from build123d import *

# Parameters (mm, degrees)
SKETCH_1_W                 = 140
SKETCH_1_H                 = 120
SKETCH_1_R                 = 11.5
EXTRUDE_1_DEPTH            = 4
SKETCH_31_R                = 2.05
SKETCH_31_R_2              = 2.1
CUT_EXTRUDE_16_DEPTH       = 10
MIRROR_2_COPY_1_SKETCH_R   = 2.05
MIRROR_2_COPY_1_SKETCH_R_2 = 2.1
MIRROR_2_COPY_1_DEPTH      = 10
FILLET_8_R                 = 25
SKETCH_32_R                = 2.1
CUT_EXTRUDE_17_DEPTH       = 10
SKETCH_33_R                = 1.6
CUT_EXTRUDE_18_DEPTH       = 10


with BuildPart() as part:
    # 草图1 → 凸台-拉伸1 (new body)
    with BuildSketch(Plane.XY):
        with Locations((70, 60)):
            Rectangle(SKETCH_1_W, SKETCH_1_H)
        with Locations((70, 60)):
            Circle(SKETCH_1_R, mode=Mode.SUBTRACT)
    extrude(amount=EXTRUDE_1_DEPTH)

    # 草图31 → 切除-拉伸16 (cut)
    with BuildSketch(Plane.XY.offset(4)):
        with Locations((9, 60)):
            Circle(SKETCH_31_R)
        with Locations((9, 88)):
            Circle(SKETCH_31_R_2)
    cut_extrude_16 = extrude(amount=-CUT_EXTRUDE_16_DEPTH, mode=Mode.SUBTRACT)

    # 镜向1: 切除-拉伸16 across plane
    add(cut_extrude_16.mirror(Plane.ZX.offset(60)), mode=Mode.SUBTRACT)

    # 镜向2: 切除-拉伸16 across plane
    add(cut_extrude_16.mirror(Plane.ZY.offset(-70)), mode=Mode.SUBTRACT)

    # 镜向2 copy 1 sketch → 镜向2 copy 1 (cut)
    with BuildSketch(Plane(origin=(140, 120, 4), x_dir=(-1, 0, 0), z_dir=(0, 0, 1))):
        with Locations((9, 60)):
            Circle(MIRROR_2_COPY_1_SKETCH_R)
        with Locations((9, 88)):
            Circle(MIRROR_2_COPY_1_SKETCH_R_2)
    extrude(amount=-MIRROR_2_COPY_1_DEPTH, mode=Mode.SUBTRACT)

    # 圆角8
    fillet_8_edges = [part.edges().sort_by_distance(p)[0] for p in [
        (0, 120, 2),
        (140, 120, 2),
        (140, 0, 2),
        (0, 0, 2),
    ]]
    fillet(fillet_8_edges, radius=FILLET_8_R)

    # 草图32 → 切除-拉伸17 (cut)
    with BuildSketch(Plane.XY.offset(4)):
        with Locations((70, 112.5)):
            Circle(SKETCH_32_R)
        with Locations((107.123106012, 97.123106012)):
            Circle(SKETCH_32_R)
        with Locations((122.5, 60)):
            Circle(SKETCH_32_R)
        with Locations((107.123106012, 22.876893988)):
            Circle(SKETCH_32_R)
        with Locations((70, 7.5)):
            Circle(SKETCH_32_R)
        with Locations((32.876893988, 22.876893988)):
            Circle(SKETCH_32_R)
        with Locations((17.5, 60)):
            Circle(SKETCH_32_R)
        with Locations((32.876893988, 97.123106012)):
            Circle(SKETCH_32_R)
    extrude(amount=-CUT_EXTRUDE_17_DEPTH, mode=Mode.SUBTRACT)

    # 草图33 → 切除-拉伸18 (cut)
    with BuildSketch(Plane.XY.offset(4)):
        with Locations((70, 80)):
            Circle(SKETCH_33_R)
        with Locations((87.320508076, 50)):
            Circle(SKETCH_33_R)
        with Locations((52.679491924, 50)):
            Circle(SKETCH_33_R)
    extrude(amount=-CUT_EXTRUDE_18_DEPTH, mode=Mode.SUBTRACT)


solid = part.part
For this review, take the finished solid that the model builds, in its own axes (mm). Round coordinates to 2 decimals unless told otherwise and drop trailing zeros. Order: outer loops, then holes, each group sorted by start corner. A loop starts at its lowest first (then second) coordinate and runs counter-clockwise, first axis right, second up. Notation, with made-up numbers: M 80.5,-19 L 124.5,-19 A18 ccw 124.5,-12 Z; hole C 81.25,30.25 d9. An arc over 180 degrees is marked long. Use a Markdown table: item, result. Add a question column.
Item 1: Add section A-A, the plane y = 88. Give the boundary of the cut face in (x, z), then the cut area to 3 significant figures.
Item 2: Add section D-D, the plane x = 9. Give the boundary of the cut face in (y, z).
Item 3: Mouldability with a two-part tool opening along X and no side actions: class faces 1 (the cylindrical face through (69.54, 110.45, 2.03)), 2 (the flat face through (140, 60, 2)), 3 (the flat face through (69, 48, 0)) as released by +X, released by -X, zero draft, split by the parting line, or undercut.
Item 4: Insertion check: pin 1 (5 mm diameter, centred on x = 131, y = 88, fed in from -Z); pin 2 (2.5 mm diameter, centred on x = 131, y = 60, fed in from +Z). Each pin has a flat end and moves straight along its axis. Give the tip position at first contact, or say it passes through.
Item 5: Add section C-C, the plane y = 50. Give the boundary of the cut face in (x, z), then the cut area to 3 significant figures.
Item 6: Add section B-B, the plane x = 66. Give the boundary of the cut face in (y, z).
Item 7: To check wall thickness, follow line 1 along Y through (x, z) = (70, 2.25); line 2 along Y through (x, z) = (9, 1.85); line 3 along X through (y, z) = (59.5, 0.7). State the ranges of each line that lie inside material, in increasing order.
Geometry results:
| question | item | result |
|---|---|---|
| 1 | outline | M 0,0 L 6.9,0 L 6.9,4 L 0,4 Z; M 11.1,0 L 128.9,0 L 128.9,4 L 11.1,4 Z; M 133.1,0 L 140,0 L 140,4 L 133.1,4 Z |
| 1 | area | 526 mm² |
| 2 | outline | M 5.79,0 L 29.9,0 L 29.9,4 L 5.79,4 Z; M 34.1,0 L 57.95,0 L 57.95,4 L 34.1,4 Z; M 62.05,0 L 85.9,0 L 85.9,4 L 62.05,4 Z; M 90.1,0 L 114.21,0 L 114.21,4 L 90.1,4 Z |
| 3 | face 1 | undercut |
| 3 | face 2 | released by +X |
| 3 | face 3 | zero draft |
| 4 | pin 1 | stops at z = 0 |
| 4 | pin 2 | passes through |
| 5 | outline | M 0,0 L 51.08,0 L 51.08,4 L 0,4 Z; M 54.28,0 L 64.32,0 L 64.32,4 L 54.28,4 Z; M 75.68,0 L 85.72,0 L 85.72,4 L 75.68,4 Z; M 88.92,0 L 140,0 L 140,4 L 88.92,4 Z |
| 5 | area | 489 mm² |
| 6 | outline | M 0,0 L 49.22,0 L 49.22,4 L 0,4 Z; M 70.78,0 L 120,0 L 120,4 L 70.78,4 Z |
| 7 | line 1 | y = 0 to 5.4, 9.6 to 48.5, 71.5 to 78.4, 81.6 to 110.4, 114.6 to 120 |
| 7 | line 2 | y = 5.79 to 29.9, 34.1 to 57.95, 62.05 to 85.9, 90.1 to 114.21 |
| 7 | line 3 | x = 0 to 7.01, 10.99 to 15.46, 19.54 to 58.51, 81.49 to 120.46, 124.54 to 129.01, 132.99 to 140 |
